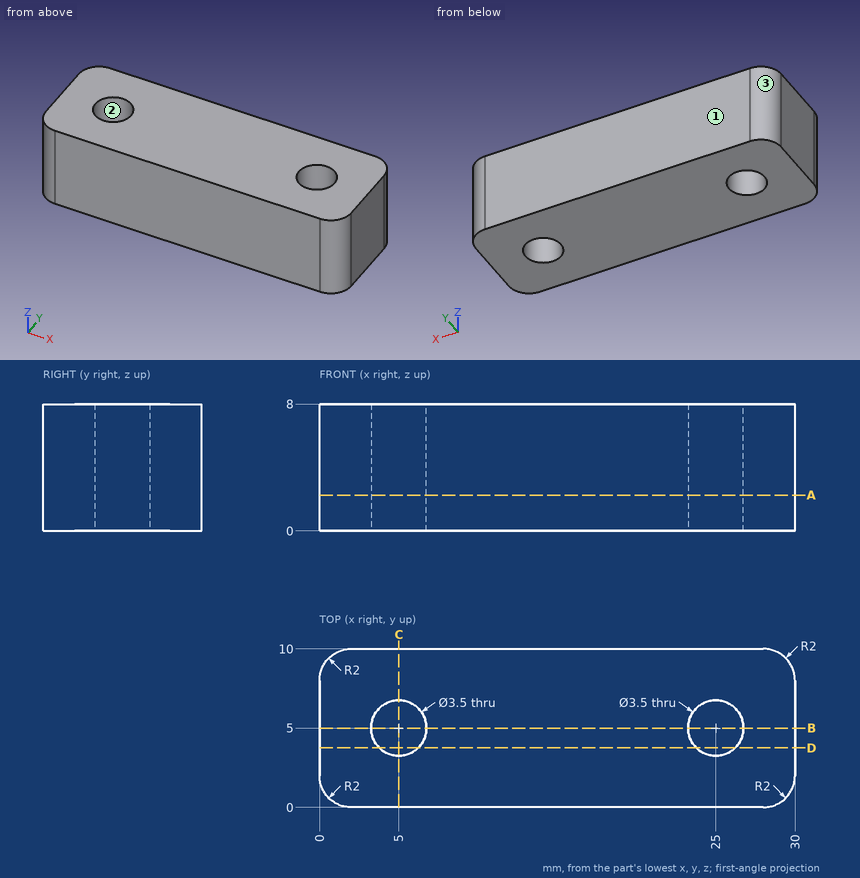
Here's the drawing with two shaded views (mm, measured from the low corner). I have some questions. Round coordinates to 2 decimals unless told otherwise and drop trailing zeros. Loops run counter-clockwise (first coordinate to the right, second up) from the corner with the lowest first, then second, coordinate; pieces in that order, holes last.
Item 1: Suppose I cut it at C-C, the plane x = 5. Write out the boundary of the cut face in (y, z), then the cut area to 3 significant figures.
Item 2: If we mould it in two halves opening along X, with no side actions, what happens to the marked faces 1, 2 and 3? For each: +X half, -X half, draft (parallel to the pull), parting line (faces both ways), or undercut.
Item 3: Suppose I cut it at B-B, the plane y = 5. Write out the boundary of the cut face in (x, z), then the cut area to 3 significant figures.
Item 4: Suppose I cut it at A-A, the plane z = 2.25. Write out the boundary of the cut face in (x, y).
Item 5: Suppose I cut it at D-D, the plane y = 3.75. Write out the boundary of the cut face in (x, z), then the cut area to 3 significant figures.
Item 6: Please list where these lines run through material, in increasing order: L1, parallel to X at y = 5, z = 4; L2, parallel to Y at x = 5, z = 3.25; L3, parallel to X at y = 4.25, z = 1.
Reported:
1. outline: (0, 0) - (3.25, 0) - (3.25, 8) - (0, 8) - close; (6.75, 0) - (10, 0) - (10, 8) - (6.75, 8) - close
1. area: 52.0 mm2
2. face 1: draft
2. face 2: undercut
2. face 3: -X half
3. outline: (0, 0) - (3.25, 0) - (3.25, 8) - (0, 8) - close; (6.75, 0) - (23.25, 0) - (23.25, 8) - (6.75, 8) - close; (26.75, 0) - (30, 0) - (30, 8) - (26.75, 8) - close
3. area: 184 mm2
4. outline: (0, 2) arc R2 ccw to (2, 0) - (28, 0) arc R2 ccw to (30, 2) - (30, 8) arc R2 ccw to (28, 10) - (2, 10) arc R2 ccw to (0, 8) - close; hole circle Ø3.5 at (5, 5); hole circle Ø3.5 at (25, 5)
5. outline: (0, 0) - (3.78, 0) - (3.78, 8) - (0, 8) - close; (6.22, 0) - (23.78, 0) - (23.78, 8) - (6.22, 8) - close; (26.22, 0) - (30, 0) - (30, 8) - (26.22, 8) - close
5. area: 201 mm2
6. L1: x = 0 to 3.25, 6.75 to 23.25, 26.75 to 30
6. L2: y = 0 to 3.25, 6.75 to 10
6. L3: x = 0 to 3.42, 6.58 to 23.42, 26.58 to 30
